Answer from the drawing. Dimensions are ordinates in mm from the lowest x, y and z of the part. A direction names the side the tool comes from. Give positions to 0.01 mm unless a question says otherwise; leave off trailing zeros. Loops run counter-clockwise (first coordinate to the right, second up) from the corner with the lowest first, then second, coordinate; pieces in that order, holes last. Notation, with made-up numbers: (84.25, 56) - (106.25, 56) arc R26 ccw to (106.25, 74) - close; hole circle Ø1 at (81.5, 18). An arc over 180 degrees is marked (long way). Write each question's results on one line, items separated by ' | '. Start each with the question number.
Q1. For the marked faces 4, 5, 6 and 7, determine the directions among +Z, -Z, +X, -X, +Y, -Y from which every point of the face is accessible in a straight line to the end or side of a thin tool.
Q2. The part is cut by section C-C, the plane z = 3.5. Write down the section's boundary in (x, y), plus the area to 3 significant figures.
Q3. Given pin 1 (7.5 mm diameter, centred on x = 47, z = 8, fed in from +Y); pin 2 (3 mm diameter, centred on x = 12, z = 4.5, fed in from +Y); pin 3 (4 mm diameter, centred on x = 48.5, z = 7, fed in from -Y); pin 4 (2 mm diameter, centred on x = 11.5, z = 5, fed in from -Y), each flat-ended and moving along its own axis, determine where each tip first touches the part or whether it passes through.
Q4. The part is cut by section B-B, the plane z = 8. Write down the section's boundary in (x, y), plus the area to 3 significant figures.
Q5. The part is cut by section D-D, the plane y = 8.75. Write down the section's boundary in (x, z) (1 decimal), plus the area to 3 significant figures.
Q6. Determine the mould class of the marked faces 1, 2 and 3 for opening direction X: +X half, -X half, draft (parallel to the pull), parting line (faces both ways), or undercut.
Q7. The part is cut by section A-A, the plane x = 47. Write down the section's boundary in (y, z).
Q8. Find the intervals of material crossed by line 1 (Z direction, x = 4, y = 15.8); line 2 (Y direction, x = 46.5, z = 12.25); line 3 (X direction, y = 15, z = 11.5), in increasing order. Write a range as from..to.
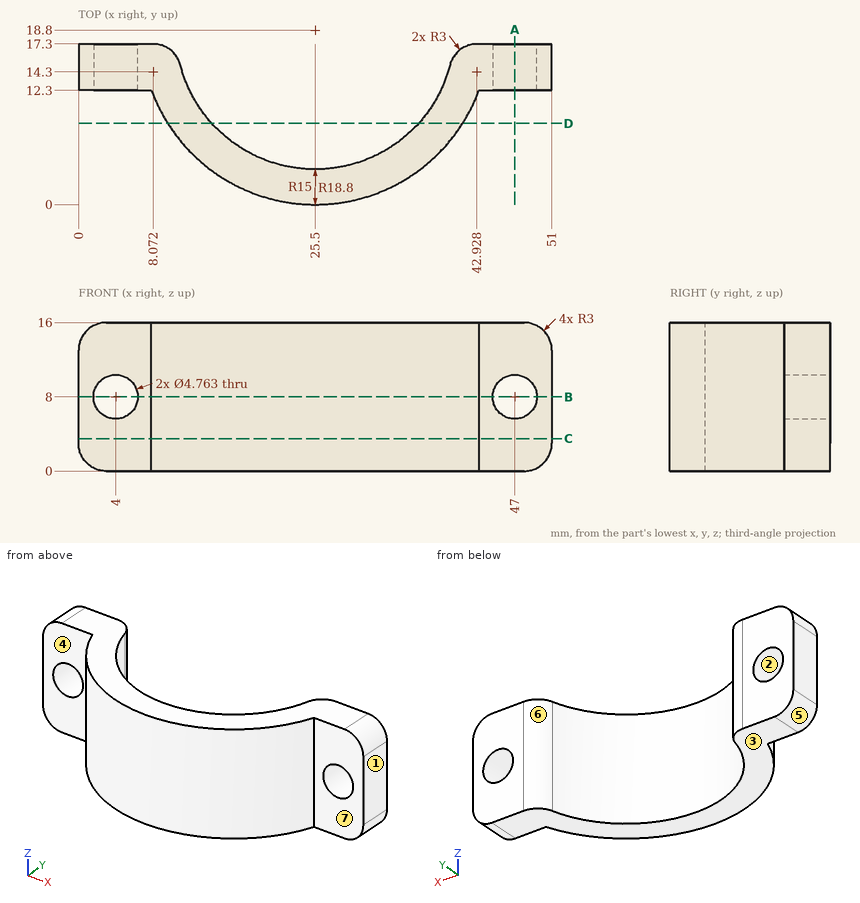
Check sheet entries:
1) face 4: +Z, -Z, -X, -Y | face 5: -Z, -X, +Y, -Y | face 6: +Z, -Z, +Y | face 7: +Z, -Z, +X, -Y
2) outline: (0, 12.3) - (7.86, 12.3) arc R18.8 ccw to (43.14, 12.3) - (51, 12.3) - (51, 17.3) - (42.93, 17.3) arc R3 ccw to (40.02, 15.05) arc R15 cw to (10.98, 15.05) arc R3 ccw to (8.07, 17.3) - (0, 17.3) - close | area: 260 mm^2
3) pin 1: stops at y = 17.3 | pin 2: stops at y = 16.06 | pin 3: stops at y = 12.3 | pin 4: stops at y = 5.22
4) outline: (0, 12.3) - (1.62, 12.3) - (1.62, 17.3) - (0, 17.3) - close; (6.38, 12.3) - (7.86, 12.3) arc R18.8 ccw to (43.14, 12.3) - (44.62, 12.3) - (44.62, 17.3) - (42.93, 17.3) arc R3 ccw to (40.02, 15.05) arc R15 cw to (10.98, 15.05) arc R3 ccw to (8.07, 17.3) - (6.38, 17.3) - close; (49.38, 12.3) - (51, 12.3) - (51, 17.3) - (49.38, 17.3) - close | area: 212 mm^2
5) outline: (9.6, 0) - (14.4, 0) - (14.4, 16) - (9.6, 16) - close; (36.6, 0) - (41.4, 0) - (41.4, 16) - (36.6, 16) - close | area: 152 mm^2
6) face 1: +X half | face 2: undercut | face 3: draft
7) outline: (12.3, 0) - (17.3, 0) - (17.3, 5.62) - (12.3, 5.62) - close; (12.3, 10.38) - (17.3, 10.38) - (17.3, 16) - (12.3, 16) - close
8) line 1: z = 0..5.62, 10.38..16 | line 2: y = 12.3..17.3 | line 3: x = 0..10.99, 40.01..51
